Here's how the part is built. I have some questions about the finished solid (model axes, mm). A direction names the side the tool comes from. Give positions to 0.01 mm unless a question says otherwise; leave off trailing zeros. Write each loop counter-clockwise with the first axis right and the second up, starting at its lowest first coordinate (ties: lowest second). Pieces come first, ordered by that corner, then holes. Notation, with made-up numbers: (30, 75.25) - (80, 75.25) arc R21 cw to (80, 102.25) - close; hole circle Ø6 at (4.25, -36.75). An arc over 180 degrees is marked (long way). Use a Markdown table: item, result.
```python
from build123d import *

# Parameters (mm, degrees)
SKETCH1_W           = 1
SKETCH1_H           = 25
BOSS_EXTRUDE1_DEPTH = 9.5
SKETCH2_W           = 1
SKETCH2_H           = 1
BOSS_EXTRUDE2_DEPTH = 9.5


with BuildPart() as part:
    # Sketch1 → Boss-Extrude1 (new body)
    with BuildSketch(Plane(origin=(0, 0, 0), x_dir=(1, 0, 0), z_dir=(0, 1, 0))):
        with Locations((-0.5, 12.5)):
            Rectangle(SKETCH1_W, SKETCH1_H)
        Polygon((-1, 22.5), (-1, 25), (-1.75, 22.5), align=None)
        Polygon((-1, 20), (-1, 22.5), (-1.75, 20), align=None)
        Polygon((-1, 17.5), (-1, 20), (-1.75, 17.5), align=None)
        Polygon((-1, 15), (-1, 17.5), (-1.75, 15), align=None)
        Polygon((-1, 12.5), (-1, 15), (-1.75, 12.5), align=None)
        Polygon((-1.75, 10), (-1, 10), (-1, 12.5), align=None)
        Polygon((-1.75, 7.5), (-1, 7.5), (-1, 10), align=None)
        Polygon((-1.75, 5), (-1, 5), (-1, 7.5), align=None)
        Polygon((-1.75, 0), (-1, 0), (-1, 2.5), align=None)
        Polygon((-1.75, 2.5), (-1, 2.5), (-1, 5), align=None)
    extrude(amount=BOSS_EXTRUDE1_DEPTH)

    # Sketch2 → Boss-Extrude2 (add)
    with BuildSketch(Plane(origin=(0, 9.5, 0), x_dir=(1, 0, 0), z_dir=(0, 1, 0))):
        with Locations((0.5, 12.5)):
            Rectangle(SKETCH2_W, SKETCH2_H)
    extrude(amount=-BOSS_EXTRUDE2_DEPTH)


solid = part.part
```
Item 1: For faces 5 (the flat face through (0, 5, -6)), 6 (the flat face through (-1, 9.5, -13)), 7 (the flat face through (1, 4.8, -12.5)), 8 (the flat face through (-1.37, 4.68, -18.77)), 9 (the flat face through (0.5, 4.8, -13)), which set-ups out of +Z, -Z, +X, -X, +Y, -Y let a thin tool reach every point of the face, with its end or its side?
Values:
| item | result |
|---|---|
| face 5 | +Z, +X, +Y, -Y |
| face 6 | +Z, -Z, +X, -X, +Y |
| face 7 | +Z, -Z, +X, +Y, -Y |
| face 8 | -X, +Y, -Y |
| face 9 | -Z, +X, +Y, -Y |
Item 2: Thinking about a two-plate mould opening in Z: for faces 1 (the flat face through (-1, 0, -13)), 2 (the flat face through (-1.37, 4.68, -21.27)), 3 (the flat face through (-1, 5, 0)), 4 (the flat face through (-0.5, 4.7, -25)), which applies, +Z half, -Z half, draft (parallel to the pull), parting line (faces both ways), or undercut?
Values:
| item | result |
|---|---|
| face 1 | draft |
| face 2 | undercut |
| face 3 | +Z half |
| face 4 | -Z half |
Item 3: Will these pins go through, and if not, where does the flat tip stop? pin 1 Ø0.6 at (x, y) = (-1.5, 4) entering from +Z; pin 2 Ø3 at (y, z) = (5.5, -6) entering from +X; pin 3 Ø0.8 at (x, y) = (0.5, 7) entering from -Z; pin 4 Ø0.5 at (x, y) = (0.5, 5.5) entering from +Z.
Values:
| item | result |
|---|---|
| pin 1 | stops at z = 0 |
| pin 2 | stops at x = 0 |
| pin 3 | stops at z = -13 |
| pin 4 | stops at z = -12 |
Item 4: If we section it at C-C, the plane x = 0.6: Write out the boundary of the cut face in (y, z), plus the area to 3 significant figures.
Values:
| item | result |
|---|---|
| outline | (0, -13) - (9.5, -13) - (9.5, -12) - (0, -12) - close |
| area | 9.50 mm2 |
Item 5: If we section it at B-B, the plane z = -13.5: Write out the boundary of the cut face in (x, y), plus the area to 3 significant figures.
Values:
| item | result |
|---|---|
| outline | (-1.45, 0) - (0, 0) - (0, 9.5) - (-1.45, 9.5) - close |
| area | 13.8 mm2 |
Item 6: I need wall thicknesses on line 1 along Z through (x, y) = (0.25, 5); line 2 along X through (y, z) = (0.5, -18.75) (3 decimals); line 3 along X through (y, z) = (9.25, -5.25) (3 decimals). Which ranges of each line are inside material? Lowest first, please. Write a range as [from, to].
Values:
| item | result |
|---|---|
| line 1 | z = [-13, -12] |
| line 2 | x = [-1.375, 0] |
| line 3 | x = [-1.675, 0] |
Item 7: If we section it at A-A, the plane y = 2.5: Write out the boundary of the cut face in (x, z), plus the area to 3 significant figures.
Values:
| item | result |
|---|---|
| outline | (-1.75, -22.5) - (-1, -25) - (0, -25) - (0, -13) - (1, -13) - (1, -12) - (0, -12) - (0, 0) - (-1.75, 0) - (-1, -2.5) - (-1.75, -2.5) - (-1, -5) - (-1.75, -5) - (-1, -7.5) - (-1.75, -7.5) - (-1, -10) - (-1.75, -10) - (-1, -12.5) - (-1.75, -12.5) - (-1, -15) - (-1.75, -15) - (-1, -17.5) - (-1.75, -17.5) - (-1, -20) - (-1.75, -20) - (-1, -22.5) - close |
| area | 35.4 mm2 |
